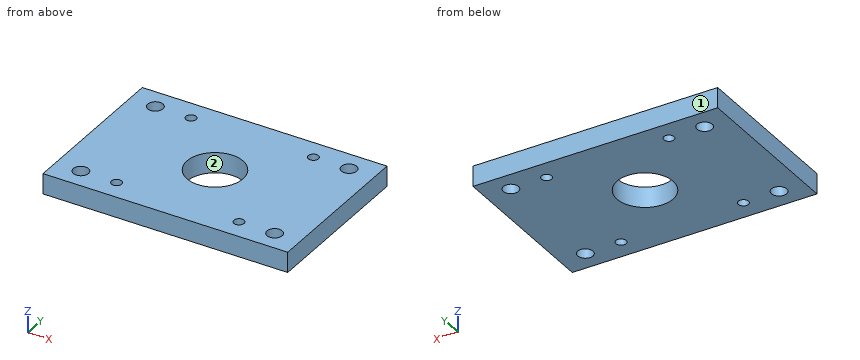
```python
from build123d import *

# Parameters (mm, degrees)
SKETCH1_W               = 76.2
SKETCH1_H               = 50.8
BOSS_EXTRUDE1_DEPTH     = 6.35
SKETCH3_R               = 2.38125
CUT_EXTRUDE6_DEPTH      = 7.35
MIRROR2_COPY_1_SKETCH_R = 2.38125
MIRROR2_COPY_1_DEPTH    = 7.35
SKETCH2_R               = 8.73125
CUT_EXTRUDE7_DEPTH      = 7.35
SKETCH5_R               = 1.5875
CUT_EXTRUDE8_DEPTH      = 7.35


with BuildPart() as part:
    # Sketch1 → Boss-Extrude1 (new body)
    with BuildSketch(Plane.XY):
        with Locations((38.1, 25.4)):
            Rectangle(SKETCH1_W, SKETCH1_H)
    extrude(amount=BOSS_EXTRUDE1_DEPTH)

    # Sketch3 → Cut-Extrude6 (cut, through all)
    with BuildSketch(Plane(origin=(0, 0, 0), x_dir=(-1, 0, 0), z_dir=(0, 0, -1))):
        with Locations((-68.2625, 44.45)):
            Circle(SKETCH3_R)
    cut_extrude6 = extrude(amount=-CUT_EXTRUDE6_DEPTH, mode=Mode.SUBTRACT)

    # Mirror1: Cut-Extrude6 across plane
    add(cut_extrude6.mirror(Plane(origin=(38.1, 0, 0), x_dir=(0, 0, 1), z_dir=(1, 0, 0))), mode=Mode.SUBTRACT)

    # Mirror2: Cut-Extrude6 across plane
    add(cut_extrude6.mirror(Plane(origin=(0, 25.4, 0), x_dir=(0, 0, 1), z_dir=(0, -1, 0))), mode=Mode.SUBTRACT)

    # Mirror2 copy 1 sketch → Mirror2 copy 1 (cut, through all)
    with BuildSketch(Plane(origin=(76.2, 50.8, 0), x_dir=(1, 0, 0), z_dir=(0, 0, -1))):
        with Locations((-68.2625, 44.45)):
            Circle(MIRROR2_COPY_1_SKETCH_R)
    extrude(amount=-MIRROR2_COPY_1_DEPTH, mode=Mode.SUBTRACT)

    # Sketch2 → Cut-Extrude7 (cut, through all)
    with BuildSketch(Plane(origin=(0, 0, 0), x_dir=(-1, 0, 0), z_dir=(0, 0, -1))):
        with Locations((-38.1, 25.4)):
            Circle(SKETCH2_R)
    extrude(amount=-CUT_EXTRUDE7_DEPTH, mode=Mode.SUBTRACT)

    # Sketch5 → Cut-Extrude8 (cut, through all)
    with BuildSketch(Plane(origin=(0, 0, 0), x_dir=(-1, 0, 0), z_dir=(0, 0, -1))):
        with Locations((-19.05, 44.45)):
            Circle(SKETCH5_R)
        with Locations((-19.05, 6.35)):
            Circle(SKETCH5_R)
        with Locations((-57.15, 44.45)):
            Circle(SKETCH5_R)
        with Locations((-57.15, 6.35)):
            Circle(SKETCH5_R)
    extrude(amount=-CUT_EXTRUDE8_DEPTH, mode=Mode.SUBTRACT)


solid = part.part
```
Model file for the job. Use its own axes, mm. Face numbers are marked on the shaded views. Coordinates: 2 decimals unless noted, no trailing zeros. Order: outer loops, then holes, each group sorted by start corner. A loop starts at its lowest first (then second) coordinate and runs counter-clockwise, first axis right, second up. Notation, with made-up numbers: M 34,-14 L 41,-14 A14 ccw 41,1 Z; hole C -6,23.5 d11. An arc over 180 degrees is marked long. Answer as CSV lines item,"result".
(1) Band-saw the part on B-B, the plane x = 38.1. List the corners of the cut face in (y, z), then the cut area to 3 significant figures.
Geometry says:
outline,"M 0,0 L 16.67,0 L 16.67,6.35 L 0,6.35 Z; M 34.13,0 L 50.8,0 L 50.8,6.35 L 34.13,6.35 Z"
area,"212 mm2"
(2) Band-saw the part on D-D, the plane x = 19.05. List the corners of the cut face in (y, z), then the cut area to 3 significant figures.
Geometry says:
outline,"M 0,0 L 4.76,0 L 4.76,6.35 L 0,6.35 Z; M 7.94,0 L 42.86,0 L 42.86,6.35 L 7.94,6.35 Z; M 46.04,0 L 50.8,0 L 50.8,6.35 L 46.04,6.35 Z"
area,"282 mm2"
(3) Pull direction X, two halves, no side cores. Call the marked faces 1 and 2: +X half, -X half, draft (parallel to the pull), parting line (faces both ways), or undercut.
Geometry says:
face 1,"draft"
face 2,"undercut"
(4) Band-saw the part on C-C, the plane z = 1.5. State how many separate pieces and enclosed holes the cut face has, then the cut area to 3 significant figures.
Geometry says:
separate pieces,"1"
enclosed holes,"9"
area,"3,530 mm2"
(5) Flat gauge pin, fed straight in: pin 1 (3 mm diameter, centred on y = 27, z = 4.5, fed in from -X). Where does the tip first touch, or does it go through?
Geometry says:
pin 1,"stops at x = 0"
(6) Band-saw the part on A-A, the plane y = 6.35. List the corners of the cut face in (x, z).
Geometry says:
outline,"M 0,0 L 5.56,0 L 5.56,6.35 L 0,6.35 Z; M 10.32,0 L 17.46,0 L 17.46,6.35 L 10.32,6.35 Z; M 20.64,0 L 55.56,0 L 55.56,6.35 L 20.64,6.35 Z; M 58.74,0 L 65.88,0 L 65.88,6.35 L 58.74,6.35 Z; M 70.64,0 L 76.2,0 L 76.2,6.35 L 70.64,6.35 Z"
(7) Wall check: line 1 along Y through (x, z) = (57.15, 4.75); line 2 along Y through (x, z) = (9.5, 5.25); line 3 along X through (y, z) = (5, 0.5). Give the ranges that are in metal, low to high.
Geometry says:
line 1,"y = 0 to 4.76, 7.94 to 42.86, 46.04 to 50.8"
line 2,"y = 0 to 4.55, 8.15 to 42.65, 46.25 to 50.8"
line 3,"x = 0 to 5.98, 9.9 to 18.21, 19.89 to 56.31, 57.99 to 66.3, 70.22 to 76.2"
